Autodesk Inventor part; units mm, degrees
ref_plane "YZ Plane" through (0, 0, 0) normal (1, 0, 0) x (0, 1, 0)
ref_plane "XZ Plane" through (0, 0, 0) normal (0, 1, 0) x (-1, 0, 0)
ref_plane "XY Plane" through (0, 0, 0) normal (0, 0, 1) x (1, 0, 0)
sketch "Sketch1" plane through (0, 0, 0) normal (0, 1, 0) x (-1, 0, 0)
  line L0 (-60, 60) -> (60, 60)
  line L1 (60, 60) -> (60, -60)
  line L2 (60, -60) -> (-60, -60)
  line L3 (-60, -60) -> (-60, 60)
  line L4 (-60, 60) -> (60, -60) construction
  line L5 (60, 60) -> (-60, -60) construction
  point P0 (0, 0)
  dimension "d0" = 120
  dimension "d1" = 120
extrude "Extrusion1" add sketch "Sketch1" along normal blind 5
sketch "Sketch2" plane through (0, 5, 0) normal (0, 1, 0) x (1, 0, 0)
  line L0 (55, -55) -> (-55, -55) construction
  line L1 (-55, -55) -> (-55, 55) construction
  line L2 (-55, 55) -> (55, 55) construction
  line L3 (55, 55) -> (55, -55) construction
  line L4 (55, -55) -> (-55, 55) construction
  line L5 (-55, -55) -> (55, 55) construction
  circle A0 centre (-55, 55) radius 2
  circle A1 centre (-55, -55) radius 2
  circle A2 centre (55, 55) radius 2
  circle A3 centre (55, -55) radius 2
  point P0 (0, 0)
  dimension "d4" = 110
  dimension "d5" = 110
  dimension "d6" = 4
  dimension "d7" = 4
  dimension "d8" = 4
  dimension "d9" = 4
extrude "Extrusion2" cut sketch "Sketch2" against normal blind 5
fillet "Fillet1" radius 5 4 edges at (60, 2.5, -60) (60, 2.5, 60) (-60, 2.5, -60) (-60, 2.5, 60)
sketch "Sketch4" plane through (0, 5, 0) normal (0, 1, 0) x (1, 0, 0)
  line L0 (-11.5, 7.5) -> (-7.5, 7.5)
  line L1 (-7.5, 7.5) -> (-7.5, -7.5)
  line L2 (-7.5, -7.5) -> (-11.5, -7.5)
  line L3 (-11.5, -7.5) -> (-11.5, 7.5)
  line L4 (-11.5, 7.5) -> (-7.5, -7.5) construction
  line L5 (-7.5, 7.5) -> (-11.5, -7.5) construction
  circle A0 centre (4.5, 4.25) radius 1.25
  circle A1 centre (4.5, -4.25) radius 1.25
  point P0 (0, 0)
  point P1 (-9.5, 0)
  dimension "d14" = 4
  dimension "d15" = 15
  dimension "d16" = 9.5
  dimension "d17" = 14
  dimension "d18" = 14
  dimension "d19" = 2.5
  dimension "d20" = 2.5
  dimension "d21" = 8.5
  dimension "d22" = 4.25
extrude "Extrusion3" cut sketch "Sketch4" against normal blind 10
properties part number "Calibration Arena"
Geometry check sheet. Reference: the model listing, model coordinates, mm. A direction names the side the tool comes from. Round coordinates to 2 decimals unless told otherwise and drop trailing zeros. Order: outer loops, then holes, each group sorted by start corner. A loop starts at its lowest first (then second) coordinate and runs counter-clockwise, first axis right, second up. Notation, with made-up numbers: (8.5, -33) - (54.5, -33) arc R11 cw to (54.5, -25) - close; hole circle Ø11 at (86, 48.25). An arc over 180 degrees is marked (long way). Use a Markdown table: item, result. Add a question column.
1) Section check A-A (x = -10). Record the cut outline in (y, z), then the cut area to 3 significant figures.
2) Thickness scan on line 1 along X through (y, z) = (2.9, 55); line 2 along X through (y, z) = (1.25, -4.25). Record the ranges inside material, lowest first.
3) Mould release check, pull along X, two halves, no side actions. Record for faces 1 (the cylindrical face through (58, 3, 59)), 2 (the flat face through (-1, 2, -60)), 3 (the flat face through (-7.5, 3, 0)): released by +X, released by -X, zero draft, split by the parting line, or undercut.
4) Set-up check for faces 4 (the flat face through (-11.5, 3, 0)), 5 (the flat face through (-60, 2, 1)): record each of +Z, -Z, +X, -X, +Y, -Y from which the full face is reachable in a straight line by a thin tool's end or side.
Established:
| question | item | result |
|---|---|---|
| 1 | outline | (0, -60) - (5, -60) - (5, -7.5) - (0, -7.5) - close; (0, 7.5) - (5, 7.5) - (5, 60) - (0, 60) - close |
| 1 | area | 525 mm2 |
| 2 | line 1 | -60 to -57, -53 to 53, 57 to 60 |
| 2 | line 2 | -60 to -11.5, -7.5 to 3.25, 5.75 to 60 |
| 3 | face 1 | released by +X |
| 3 | face 2 | zero draft |
| 3 | face 3 | undercut |
| 4 | face 4 | +Y, -Y |
| 4 | face 5 | +Z, -Z, -X, +Y, -Y |
